For this review, use the dimensioned drawing (mm, ordinates from the lowest corner) and the shaded views. A direction names the side the tool comes from. Round coordinates to 2 decimals unless told otherwise and drop trailing zeros. Write each loop counter-clockwise with the first axis right and the second up, starting at its lowest first coordinate (ties: lowest second). Pieces come first, ordered by that corner, then holes. Notation, with made-up numbers: M -0.5,81 L 34.5,81 A34 ccw 34.5,115 Z; hole C 88.5,84 d10. An arc over 180 degrees is marked long. Use one line per item in the form item = value. Start each with the question number.
Item 1: For the marked faces 1 and 2, list the 3-axis set-ups (+Z, -Z, +X, -X, +Y, -Y) from which the entire face can be reached by the end or side of a thin tool; tool diameter is ignored.
Item 2: For line 1 (Z direction, x = 25, y = 40.5); line 2 (Z direction, x = 23.5, y = 21); line 3 (X direction, y = 27, z = 27.5) (1 decimal), list the stretches that pass through material, from the lowest coordinate up. Write a range as [from, to].
Item 3: Add section B-B (x = 26.5). State the section outline as (y, z) points (1 decimal), and give its area (3 significant figures).
Item 4: For P1, Ø5, axis at y = 42.5, z = 20, coming from the +X side; P2, Ø8, axis at x = 37, z = 23, coming from the -Y side; P3, Ø12, axis at x = 24.5, y = 47.5, coming from the -Z side; P4, Ø17.5, axis at x = 17, y = 21.5, coming from the +Z side, all flat-tipped, find the tip position at first contact; note any pin that passes through.
Item 5: Add section D-D (y = 13.5). State the section outline as (x, z) points.
Item 6: Add section A-A (y = 34). State the section outline as (x, z) points.
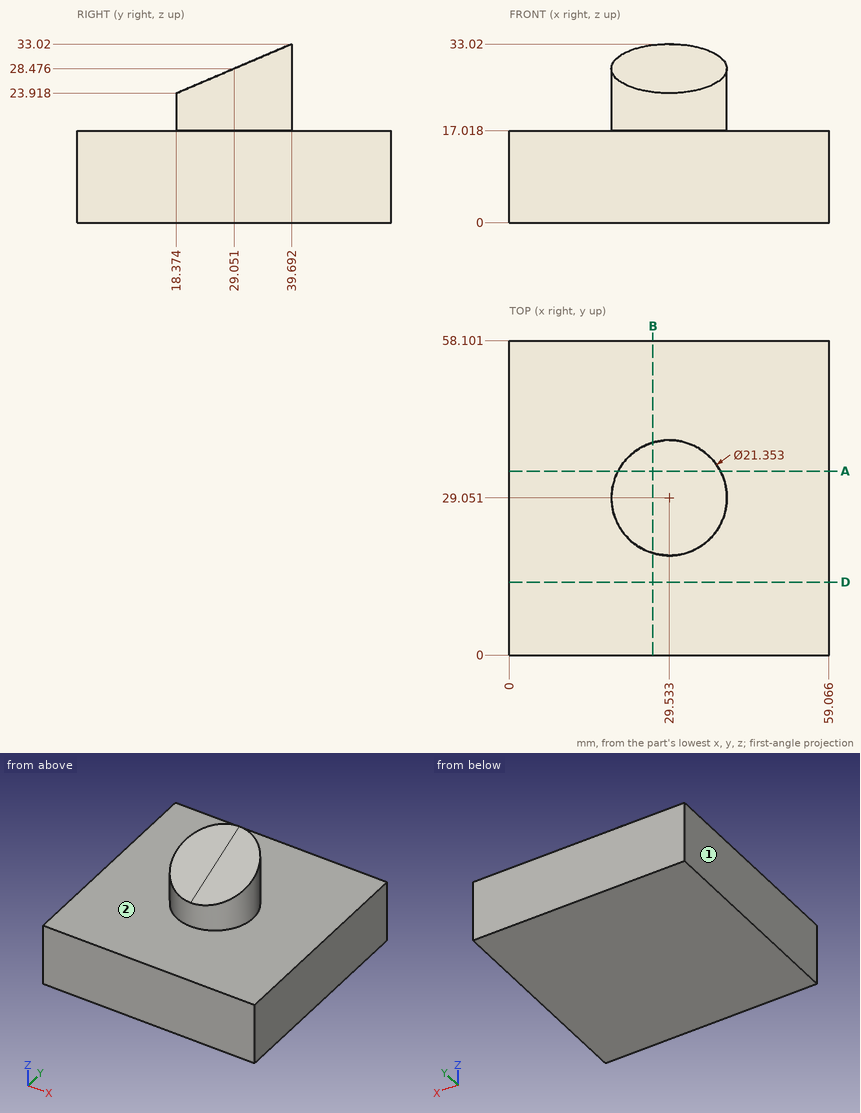
Calculated:
q1.face_1 = +Z, -Z, -X, +Y, -Y
q1.face_2 = +Z
q2.line_1 = [0, 17.02]
q2.line_2 = [0, 25.04]
q2.line_3 = [19.1, 40]
q3.outline = M 0,0 L 58.1,0 L 58.1,17 L 39.3,17 L 39.3,32.8 L 18.8,24.1 L 18.8,17 L 0,17 Z
q3.area = 1,220 mm^2
q4.P1 = through
q4.P2 = 18.95
q4.P3 = 0
q4.P4 = 28.9
q5.outline = M 0,0 L 59.07,0 L 59.07,17.02 L 0,17.02 Z
q6.outline = M 0,0 L 59.07,0 L 59.07,17.02 L 38.99,17.02 L 38.99,30.59 L 20.07,30.59 L 20.07,17.02 L 0,17.02 Z
